Part model, mm, in its own coordinate system. A direction names the side the tool comes from. Give positions to 0.01 mm unless a question says otherwise; leave off trailing zeros. Write each loop counter-clockwise with the first axis right and the second up, starting at its lowest first coordinate (ties: lowest second). Pieces come first, ordered by that corner, then holes. Notation, with made-up numbers: (56, 4) - (83, 4) arc R33 ccw to (83, 35) - close; hole circle Ø8 at (75.5, 36). An arc over 180 degrees is marked (long way). Answer in a Markdown table with one row per item. Add a question column.
1. Which spindle directions (+Z, -Z, +X, -X, +Y, -Y) get a long thin tool onto all of the face, cutting with end or side? Do faces 1 (the flat face through (0, 0, -15.875)), 2 (the flat face through (5, 0, 0)), 3 (the cylindrical face through (-3.78, -2.9, 7.13)). Say none if no direction does.
2. Probe line 1 along Z through (x, y) = (-3, -4.5); line 2 along Z through (x, y) = (-3.5, -4.5); line 3 along X through (y, z) = (5.5, 1). List the from-to ranges inside material, lowest first.
3. Band-saw the part on B-B on z = 3.25. Write the cut outline in (x, y).
4. Band-saw the part on D-D on x = 5.25. Write the cut outline in (y, z), plus the area to 3 significant figures.
5. Drop flat-ended pins along their axis: pin 1 Ø1.5 at (y, z) = (-2, -7) entering from -X; pin 2 Ø5 at (x, z) = (-1, -4) entering from -Y; pin 3 Ø3 at (x, z) = (-2.5, -3) entering from -Y. Give the stop position or say it passes through.
```python
from build123d import *

# Parameters (mm, degrees)
F1_DEPTH = 4.7625
F2_R     = 4.7625
F3_DEPTH = 15.875
F4_R     = 5.55625
F5_DEPTH = 1.5875
F6_R     = 4.7625
F7_DEPTH = 1.5875


with BuildPart() as f1:
    # F0 (on Top) → F1 (new body)
    with BuildSketch(Plane.XY):
        Polygon((-3.6661742094, -6.35), (3.6661742094, -6.35), (7.3323484187, 0), (3.6661742094, 6.35), (-3.6661742094, 6.35), (-7.3323484187, 0), align=None)
    extrude(amount=F1_DEPTH)

    # F2 (on Top) → F3 (join)
    with BuildSketch(Plane.XY):
        Circle(F2_R)
    extrude(amount=-F3_DEPTH)

    # F4 (on face) → F5 (join)
    with BuildSketch(Plane.XY.offset(4.7625)):
        Circle(F4_R)
    extrude(amount=F5_DEPTH)

    # F6 (on face) → F7 (join)
    with BuildSketch(Plane.XY.offset(6.35)):
        Circle(F6_R)
    extrude(amount=F7_DEPTH)


solid = f1.part
```
Values:
| question | item | result |
|---|---|---|
| 1 | face 1 | -Z, +X, -X, +Y, -Y |
| 1 | face 2 | -Z |
| 1 | face 3 | +Z |
| 2 | line 1 | z = 0 to 6.35 |
| 2 | line 2 | z = 0 to 4.76 |
| 2 | line 3 | x = -4.16 to 4.16 |
| 3 | outline | (-7.33, 0) - (-3.67, -6.35) - (3.67, -6.35) - (7.33, 0) - (3.67, 6.35) - (-3.67, 6.35) - close |
| 4 | outline | (-3.61, 0) - (3.61, 0) - (3.61, 4.76) - (1.82, 4.76) - (1.82, 6.35) - (-1.82, 6.35) - (-1.82, 4.76) - (-3.61, 4.76) - close |
| 4 | area | 40.1 mm² |
| 5 | pin 1 | stops at x = -4.6 |
| 5 | pin 2 | stops at y = -4.76 |
| 5 | pin 3 | stops at y = -4.66 |
